Check sheet for the drawn part. Datum: minimum x, y, z corner. Units: mm. Give positions to 0.01 mm unless a question says otherwise; leave off trailing zeros. Order: outer loops, then holes, each group sorted by start corner. A loop starts at its lowest first (then second) coordinate and runs counter-clockwise, first axis right, second up.
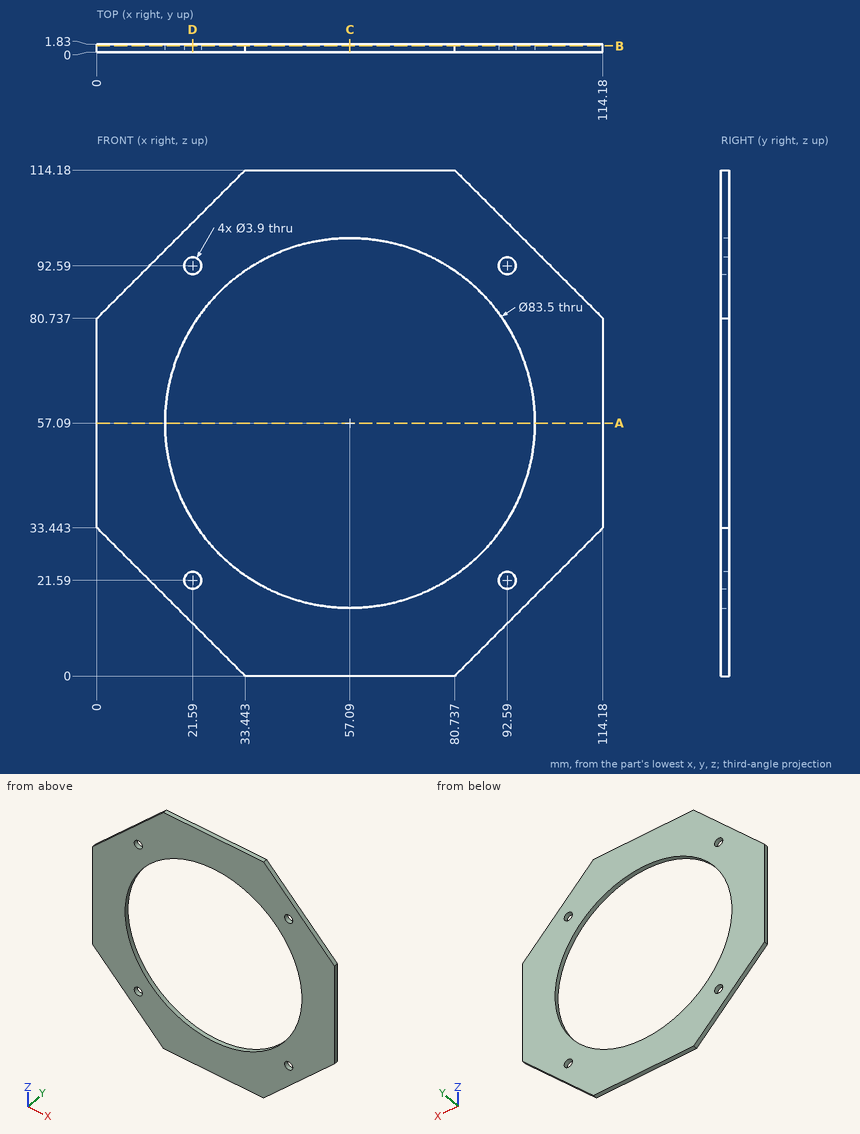
Item 1: Sectioned sample at B-B (y = 1.4). Enter the section's corners in (x, z), and give its area (3 significant figures).
Reported:
outline: (0, 33.44) - (33.44, 0) - (80.74, 0) - (114.18, 33.44) - (114.18, 80.74) - (80.74, 114.18) - (33.44, 114.18) - (0, 80.74) - close; hole circle Ø83.5 at (57.09, 57.09); hole circle Ø3.9 at (21.59, 21.59); hole circle Ø3.9 at (21.59, 92.59); hole circle Ø3.9 at (92.59, 21.59); hole circle Ø3.9 at (92.59, 92.59)
area: 5,280 mm2
Item 2: Gauge pin test, flat ends, axial feed: pin 1 (3.5 mm diameter, centred on x = 92.59, z = 21.59, fed in from +Y); pin 2 (1 mm diameter, centred on y = 1.5, z = 87.5, fed in from +X). Record the tip position at first contact, or that the pin passes through.
Reported:
pin 1: passes through
pin 2: stops at x = 107.92
Item 3: Scan lines: L1, parallel to X at y = 1.2, z = 57.09; L2, parallel to X at y = 1.55, z = 45.5; L3, parallel to Z at x = 84.5, y = 0.35 (1 decimal). Record each from-to range of solid material in increasing order.
Reported:
L1: x = 0 to 15.34, 98.84 to 114.18
L2: x = 0 to 16.98, 97.2 to 114.18
L3: z = 3.8 to 25.6, 88.6 to 110.4
Item 4: Sectioned sample at C-C (x = 57.09). Enter the section's corners in (y, z).
Reported:
outline: (0, 0) - (1.83, 0) - (1.83, 15.34) - (0, 15.34) - close; (0, 98.84) - (1.83, 98.84) - (1.83, 114.18) - (0, 114.18) - close
Item 5: Sectioned sample at D-D (x = 21.59). Enter the section's corners in (y, z).
Reported:
outline: (0, 11.85) - (1.83, 11.85) - (1.83, 19.64) - (0, 19.64) - close; (0, 23.54) - (1.83, 23.54) - (1.83, 35.12) - (0, 35.12) - close; (0, 79.06) - (1.83, 79.06) - (1.83, 90.64) - (0, 90.64) - close; (0, 94.54) - (1.83, 94.54) - (1.83, 102.33) - (0, 102.33) - close
Item 6: Sectioned sample at A-A (z = 57.09). Enter the section's corners in (x, y).
Reported:
outline: (0, 0) - (15.34, 0) - (15.34, 1.83) - (0, 1.83) - close; (98.84, 0) - (114.18, 0) - (114.18, 1.83) - (98.84, 1.83) - close
